from build123d import *

# Parameters (mm, degrees)
F0_W      = 23.5
F0_H      = 32
F1_DEPTH  = 7.75
F4_W      = 15.5
F4_H      = 5.5
F5_DEPTH  = 10.5
F1_FACE_W = 23.5
F1_FACE_H = 7.75
F5_FACE_W = 15.5
F5_FACE_H = 5.5
F7_R      = 0.9
F8_DEPTH  = 6
F9_R      = 0.6
F10_DEPTH = 140


with BuildPart() as f1:
    # F0 (on Top) → F1 (new body)
    with BuildSketch(Plane.XY):
        Rectangle(F0_W, F0_H)
    extrude(amount=F1_DEPTH)



with BuildPart() as f5:
    # F4 (on face) → F5 (new body)
    with BuildSketch(Plane(origin=(0, 16.6609531262, 1.1650473361), x_dir=(-1, 0, 0), z_dir=(0, 0.9975640503, 0.0697564737))):
        with Locations((1.6, 4.0650178096)):
            Rectangle(F4_W, F4_H)
    extrude(amount=F5_DEPTH)


with BuildPart() as f1_1:
    add(f1.part)

    add(f5.part)  # F6 merges F5
    # F1_face (on face) → F6 section 0
    with BuildSketch(Plane(origin=(0, 16, 3.875), x_dir=(-1, 0, 0), z_dir=(0, 1, 0))):
        Rectangle(F1_FACE_W, F1_FACE_H)
    # F5_face (on face) → F6 section 1
    with BuildSketch(Plane(origin=(-1.6, 16.3773918181, 5.2201629666), x_dir=(-1, 0, 0), z_dir=(0, -0.9975640503, -0.0697564737))):
        Rectangle(F5_FACE_W, F5_FACE_H)
    loft()

    # F7 (on face) → F8 (join)
    with BuildSketch(Plane.XZ.offset(16)):
        with Locations((-8.25, 6.25)):
            Circle(F7_R)
        with Locations((3.75, 6.25)):
            Circle(F7_R)
    extrude(amount=F8_DEPTH)

    # F9 (on face) → F10 (join)
    with BuildSketch(Plane.XZ.offset(22)):
        with Locations((-8.25, 6.25)):
            Circle(F9_R)
        with Locations((3.75, 6.25)):
            Circle(F9_R)
    extrude(amount=F10_DEPTH)


solid = f1_1.part
Source: CAD feature listing. Evaluate the final solid. Frame: model axes, mm. A direction names the side the tool comes from. Give positions to 0.01 mm unless a question says otherwise; leave off trailing zeros. Write each loop counter-clockwise with the first axis right and the second up, starting at its lowest first coordinate (ties: lowest second). Pieces come first, ordered by that corner, then holes. Notation, with made-up numbers: M 7,-26.75 L 28,-26.75 A19 cw 28,-22.75 Z; hole C -9,60.5 d2. An arc over 180 degrees is marked long. Return JSON: item names as keys, results as strings. Group by question number.
1) Cut plane A-A, the plane y = -24. Output: boundary loops of the cut face in (x, z).
2) Set-up query: faces 1 (the face through (0, 0, 7.75)), 2 (the face through (0, 0, 0)). Return all of +Z, -Z, +X, -X, +Y, -Y with unobstructed straight access to the full face (end or side cutting, diameter ignored); none if empty.
3) Cut plane B-B, the plane y = 0.5. Output: boundary loops of the cut face in (x, z), then the cut area to 3 significant figures.
4) Ray query, L1, parallel to Z at x = 3, y = -13; L2, parallel to X at y = -38, z = 6; L3, parallel to Y at x = 2.75, z = 5. Return the intervals inside material, ascending.
5) First-contact query: pin 1 Ø5 at (y, z) = (20.5, 6.5) entering from -X; pin 2 Ø5 at (y, z) = (-59.5, 4.5) entering from -X; pin 3 Ø1.5 at (y, z) = (-51.5, 4.5) entering from -X; pin 4 Ø4 at (x, y) = (6, -41.5) entering from +Z. Flat tips, straight axial feed; report the tip coordinate or a pass-through.
Data:
{
 "1": {"outline": "C -8.25,6.25 d1.2; C 3.75,6.25 d1.2"},
 "2": {"face 1": "+Z, +X, -X, -Y", "face 2": "-Z, +X, -X, +Y, -Y"},
 "3": {"outline": "M -11.75,0 L 11.75,0 L 11.75,7.75 L -11.75,7.75 Z", "area": "182 mm²"},
 "4": {"L1": "z = 0 to 7.75", "L2": "x = -8.8 to -7.7, 3.2 to 4.3", "L3": "y = -16 to 26.92"},
 "5": {"pin 1": "stops at x = -9.35", "pin 2": "stops at x = -8.85", "pin 3": "passes through", "pin 4": "stops at z = 6.8"}
}
